from build123d import *

# Parameters (mm, degrees)
F1_DEPTH = 20
F2_R     = 11.25
F3_DEPTH = 7
F4_R     = 6.75
F5_DEPTH = 5
F6_W     = 3
F6_H     = 32.5
F7_DEPTH = 30
F8_R     = 6.75
F9_DEPTH = 25


with BuildPart() as f1:
    # F0 (on Front) → F1 (new body, symmetric)
    with BuildSketch(Plane.XZ):
        Polygon((-25, 35), (-30, 35), (-30, 0), (1, 0), (1, 35), (-9, 35), (-9, 5), (-25, 5), align=None)
    extrude(amount=F1_DEPTH, both=True)

    # F2 (on face) → F3 (cut)
    with BuildSketch(Plane.YZ.offset(1)):
        with Locations((0, 17.5)):
            Circle(F2_R)
    extrude(amount=-F3_DEPTH, mode=Mode.SUBTRACT)

    # F4 (on face) → F5 (cut)
    with BuildSketch(Plane.YZ.offset(-6)):
        with Locations((0, 17.5)):
            Circle(F4_R)
    extrude(amount=-F5_DEPTH, mode=Mode.SUBTRACT)

    # F6 (on face) → F7 (cut)
    with BuildSketch(Plane.XY.offset(35)):
        with Locations((-26.5, 0)):
            Rectangle(F6_W, F6_H)
    extrude(amount=-F7_DEPTH, mode=Mode.SUBTRACT)

    # F8 (on face) → F9 (cut)
    with BuildSketch(Plane(origin=(-9, 0, 0), x_dir=(0, -1, 0), z_dir=(-1, 0, 0))):
        Polygon((4.1857894516, 24.75), (-4.1857894516, 24.75), (-8.3715789032, 17.5), (-4.1857894516, 10.25), (4.1857894516, 10.25), (8.3715789032, 17.5), align=None)
        with Locations((0, 17.5)):
            Circle(F8_R, mode=Mode.SUBTRACT)
        with Locations((0, 17.5)):
            Circle(F8_R)
        with BuildLine():
            ThreePointArc((4.1857894516, 24.75), (0, 25.8715789032), (-4.1857894516, 24.75))
            Line((-4.1857894516, 24.75), (4.1857894516, 24.75))
        make_face()
        with BuildLine():
            Line((-8.3715789032, 17.5), (-4.1857894516, 24.75))
            ThreePointArc((-4.1857894516, 24.75), (-7.25, 21.6857894516), (-8.3715789032, 17.5))
        make_face()
        with BuildLine():
            ThreePointArc((8.3715789032, 17.5), (7.25, 21.6857894516), (4.1857894516, 24.75))
            Line((4.1857894516, 24.75), (8.3715789032, 17.5))
        make_face()
        with BuildLine():
            Line((-4.1857894516, 10.25), (-8.3715789032, 17.5))
            ThreePointArc((-8.3715789032, 17.5), (-7.25, 13.3142105484), (-4.1857894516, 10.25))
        make_face()
        with BuildLine():
            ThreePointArc((4.1857894516, 10.25), (7.25, 13.3142105484), (8.3715789032, 17.5))
            Line((8.3715789032, 17.5), (4.1857894516, 10.25))
        make_face()
        with BuildLine():
            Line((4.1857894516, 10.25), (-4.1857894516, 10.25))
            ThreePointArc((-4.1857894516, 10.25), (0, 9.1284210968), (4.1857894516, 10.25))
        make_face()
    extrude(amount=-F9_DEPTH, mode=Mode.SUBTRACT)


solid = f1.part
Here's how the part is built. I have some questions about the finished solid (model axes, mm). A direction names the side the tool comes from. Round coordinates to 2 decimals unless told otherwise and drop trailing zeros. Order: outer loops, then holes, each group sorted by start corner. A loop starts at its lowest first (then second) coordinate and runs counter-clockwise, first axis right, second up. Notation, with made-up numbers: (46, 51.25) -> (57, 51.25) arc R33 cw to (57, 83.25) -> close; hole circle Ø8 at (36.5, 18.25). An arc over 180 degrees is marked (long way). Use CSV: the item, a comma, the result in double quotes.
1. I want a section at B-B on z = 14. List the corners of the cut face in (x, y) for me, and give its area (3 significant figures).
Recorded:
outline,"(-30, -20) -> (-25, -20) -> (-25, -16.25) -> (-28, -16.25) -> (-28, 16.25) -> (-25, 16.25) -> (-25, 20) -> (-30, 20) -> close; (-9, -20) -> (1, -20) -> (1, -10.69) -> (-6, -10.69) -> (-6, -7.6) -> (-9, -7.6) -> close; (-9, 7.6) -> (-6, 7.6) -> (-6, 10.69) -> (1, 10.69) -> (1, 20) -> (-9, 20) -> close"
area,"307 mm2"
2. Thinking about a two-plate mould opening in X: for faces 1 (the face through (-6, -2, 26)), 2 (the face through (-8, 20, 18)), 3 (the face through (-28, 0, 20)), which applies, pulls with the +X half, pulls with the -X half, needs draft (parallel to the pull), parting line crosses it, or undercut?
Recorded:
face 1,"pulls with the +X half"
face 2,"needs draft"
face 3,"undercut"
3. I'm going to push flat-ended pins straight in: P1, Ø8, axis at x = -15, z = 28, coming from the +Y side; P2, Ø6, axis at y = 2.5, z = 15, coming from the +X side; P3, Ø9.5, axis at x = -18.5, y = -3.5, coming from the +Z side. Where does each tip first touch, or does it pass through?
Recorded:
P1,"passes through"
P2,"stops at x = -28"
P3,"stops at z = 5"
4. I want a section at A-A on y = 0. List the corners of the cut face in (x, z) for me.
Recorded:
outline,"(-30, 0) -> (1, 0) -> (1, 6.25) -> (-6, 6.25) -> (-6, 9.13) -> (-9, 9.13) -> (-9, 5) -> (-28, 5) -> (-28, 35) -> (-30, 35) -> close; (-9, 25.87) -> (-6, 25.87) -> (-6, 28.75) -> (1, 28.75) -> (1, 35) -> (-9, 35) -> close"
5. I want a section at D-D on y = 14. List the corners of the cut face in (x, z) for me.
Recorded:
outline,"(-30, 0) -> (1, 0) -> (1, 35) -> (-9, 35) -> (-9, 5) -> (-28, 5) -> (-28, 35) -> (-30, 35) -> close"
6. I want a section at C-C on x = -26.5. List the corners of the cut face in (y, z) for me.
Recorded:
outline,"(-20, 0) -> (20, 0) -> (20, 35) -> (16.25, 35) -> (16.25, 5) -> (-16.25, 5) -> (-16.25, 35) -> (-20, 35) -> close"
7. Which directions (+Z, -Z, +X, -X, +Y, -Y) give clear straight access to the entire face, cutting with the end or side of a thin tool? Please do faces 4 (the face through (-2.451, -2.439, 6.518)), 5 (the face through (-27, -16.25, 20)), 6 (the face through (-25, 18, 20)).
Recorded:
face 4,"+X"
face 5,"+Z"
face 6,"+Z, +Y, -Y"
8. I need wall thicknesses on line 1 along X through (y, z) = (14.5, 23); line 2 along X through (y, z) = (-17, 22); line 3 along Z through (x, y) = (-2.5, 0). Which ranges of each line are inside material? Lowest first, please.
Recorded:
line 1,"x = -30 to -28, -9 to 1"
line 2,"x = -30 to -25, -9 to 1"
line 3,"z = 0 to 6.25, 28.75 to 35"
